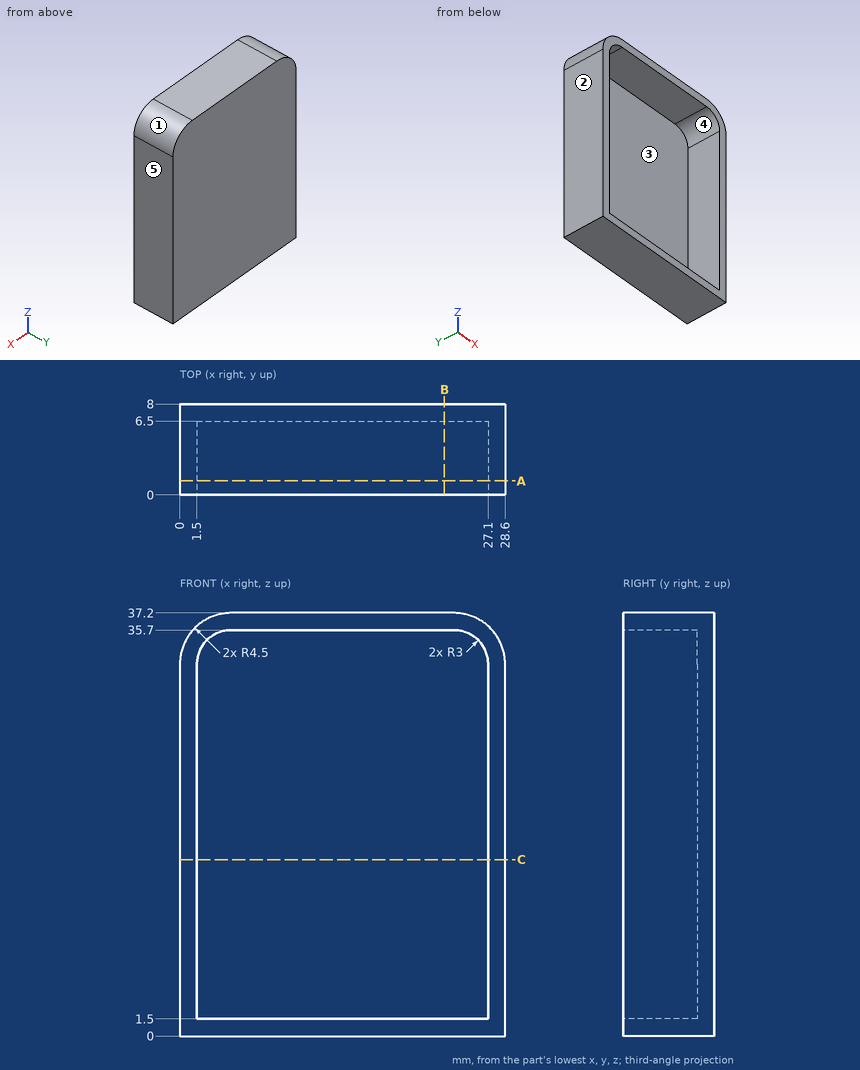
For this review, use the dimensioned drawing (mm, ordinates from the lowest corner) and the shaded views. A direction names the side the tool comes from. Round coordinates to 2 decimals unless told otherwise and drop trailing zeros. Write each loop counter-clockwise with the first axis right and the second up, starting at its lowest first coordinate (ties: lowest second). Pieces come first, ordered by that corner, then holes. Notation, with made-up numbers: (7, 45) - (15, 45) arc R27 cw to (15, 75) - close; hole circle Ø4 at (-18, 89.25). An arc over 180 degrees is marked (long way). One line per item, written item: value. Start each with the question number.
1. Clearance check with a flat-ended pin moving along its axis: P1, Ø13, axis at x = 15, z = 15.5, coming from the -Y side. State where the tip first meets the part, or that it passes through.
2. Machinability: for the marked faces 4 and 5, which of the approach directions +Z, -Z, +X, -X, +Y, -Y give a long, thin tool a straight path to every point of the face, cutting with its end or side? Answer none if there is none.
3. Consider section C-C on z = 15.5. Write out the cut boundary in (x, y).
4. The part is to be moulded in two halves that separate along X. For the marked faces 1, 2 and 3, say which applies: released by +X, released by -X, zero draft, split by the parting line, or undercut.
5. Consider section B-B on x = 23.25. Write out the cut boundary in (y, z), and give its area (3 significant figures).
6. To check wall thickness, follow L1, parallel to Z at x = 20.25, y = 2.5; L2, parallel to X at y = 3, z = 27; L3, parallel to Y at x = 4.75, z = 31.5. State the ranges of each line that lie inside material, in increasing order. Write a range as from..to.
7. Consider section A-A on y = 1.25. Write out the cut boundary in (x, z).
Checks:
1. P1: stops at y = 6.5
2. face 4: -Y
2. face 5: +Z, -Z, +X, +Y, -Y
3. outline: (0, 0) - (1.5, 0) - (1.5, 6.5) - (27.1, 6.5) - (27.1, 0) - (28.6, 0) - (28.6, 8) - (0, 8) - close
4. face 1: released by +X
4. face 2: released by -X
4. face 3: undercut
5. outline: (0, 0) - (8, 0) - (8, 37.2) - (0, 37.2) - (0, 35.7) - (6.5, 35.7) - (6.5, 1.5) - (0, 1.5) - close
5. area: 75.3 mm^2
6. L1: z = 0..1.5, 35.7..37.2
6. L2: x = 0..1.5, 27.1..28.6
6. L3: y = 6.5..8
7. outline: (0, 0) - (28.6, 0) - (28.6, 32.7) arc R4.5 ccw to (24.1, 37.2) - (4.5, 37.2) arc R4.5 ccw to (0, 32.7) - close; hole (1.5, 1.5) - (27.1, 1.5) - (27.1, 32.7) arc R3 ccw to (24.1, 35.7) - (4.5, 35.7) arc R3 ccw to (1.5, 32.7) - close
